Geometry: final body of the model. Coordinates: model frame, mm. A direction names the side the tool comes from. Round coordinates to 2 decimals unless told otherwise and drop trailing zeros. Order: outer loops, then holes, each group sorted by start corner. A loop starts at its lowest first (then second) coordinate and runs counter-clockwise, first axis right, second up. Notation, with made-up numbers: M 51.25,69 L 102.25,69 A22 cw 102.25,75 Z; hole C 83.5,65 d10. An arc over 180 degrees is marked long. Return JSON: item names as keys, results as strings. Group by question number.
Q1. Contact query for flat-ended pins moving along their axis: pin 1 (6 mm diameter, centred on y = -2.5, z = -26.5, fed in from +X); pin 2 (2.5 mm diameter, centred on x = 0.5, y = -2, fed in from +Z); pin 3 (6 mm diameter, centred on y = -3, z = -51, fed in from +X). Output: stop coordinate, or through.
Q2. Cut plane B-B on z = 4. Output: boundary loops of the cut face in (x, y) (1 decimal), and give its area (3 significant figures).
Q3. Ray query, probe 1 along Z at (x, y) = (-4.25, 9.25) (3 decimals); probe 2 along Z at (x, y) = (1, -2.75); probe 3 along X at (y, z) = (-0.25, -49.5). Return the intervals inside material, ascending.
Q4. Mould query, pull axis X, two halves, no side actions, for faces 4 (the face through (7.75, -1.72, -21.91)), 5 (the face through (0, -5, 9.525)), 6 (the face through (0, -3.962, 7)). Classes: released by +X, released by -X, zero draft, split by the parting line, or undercut.
Q5. Access query for faces 1 (the face through (10.6, -3.34, 4.7)), 2 (the face through (0, 3.962, 7)), 3 (the face through (-8, 3, 0)). Directions: +Z, -Z, +X, -X, +Y, -Y. A direction counts if a zero-diameter tool reaches every point of the face in a straight line with its end or side. Return the directions, or none.
Q6. Cut plane C-C on z = -12. Output: boundary loops of the cut face in (x, y) (1 decimal).
Solid Edge part; units mm, degrees
sketch "Sketch1" plane through (0, 0, 0) normal (0, 0, 1) x (1, 0, 0)
  circle A0 centre (0, 0) radius 11.1125
extrude "Protrusion1" add sketch "Sketch1" along normal blind 9.525
sketch "Sketch2" plane through (0, 0, 0) normal (0, 0, -1) x (0, 1, 0)
  circle A0 centre (0, 0) radius 7.9375
extrude "Protrusion2" add sketch "Sketch2" along normal blind 44.45
sketch "Sketch3" plane through (0, 0, -44.45) normal (0, 0, -1) x (0, 1, 0)
  circle A0 centre (0, 0) radius 6.35
extrude "Protrusion3" add sketch "Sketch3" along normal blind 19.05
sketch "Sketch4" plane through (0, 0, 9.525) normal (0, 0, 1) x (0, 1, 0)
  line L0 (-3.9624, 2.1791) -> (0, 4.7782)
  line L1 (-3.9624, -2.5597) -> (-3.9624, 2.1791)
  line L2 (-3.9624, -2.5597) -> (0, -4.7782)
  line L3 (3.9624, -2.5597) -> (0, -4.7782)
  line L4 (3.9624, -2.5597) -> (3.9624, 2.1791)
  line L5 (3.9624, 2.1791) -> (0, 4.7782)
extrude "Cutout1" cut sketch "Sketch4" against normal blind 4.7625
chamfer "Chamfer1" distance 0.7874 angle 45 1 edges at (0, -6.35, -63.5)
properties part number "24104955"
Result sheet:
{
 "1": {"pin 1": "stops at x = 7.94", "pin 2": "stops at z = 4.76", "pin 3": "stops at x = 6.35"},
 "2": {"outline": "C 0,0 d22.2", "area": "388 mm²"},
 "3": {"probe 1": "z = 0 to 9.525", "probe 2": "z = -63.5 to 4.76", "probe 3": "x = -6.35 to 6.35"},
 "4": {"face 4": "split by the parting line", "face 5": "zero draft", "face 6": "undercut"},
 "5": {"face 1": "+Z, -Z", "face 2": "+Z", "face 3": "-Z"},
 "6": {"outline": "C 0,0 d15.9"}
}
